Input: part model. Units: mm. Frame: model coordinates. A direction names the side the tool comes from. Give positions to 0.01 mm unless a question says otherwise; leave off trailing zeros. Order: outer loops, then holes, each group sorted by start corner. A loop starts at its lowest first (then second) coordinate and runs counter-clockwise, first axis right, second up. Notation, with made-up numbers: (67, 77) - (93, 77) arc R19 ccw to (93, 86) - close; hole circle Ø10 at (79.25, 45). An arc over 180 degrees is marked (long way). Use a Markdown table: item, result.
Autodesk Inventor part; units mm, degrees
ref_plane "YZ Plane" through (0, 0, 0) normal (1, 0, 0) x (0, 1, 0)
ref_plane "XZ Plane" through (0, 0, 0) normal (0, 1, 0) x (-1, 0, 0)
ref_plane "XY Plane" through (0, 0, 0) normal (0, 0, 1) x (1, 0, 0)
sketch "Boceto1" plane through (0, 0, 0) normal (0, 0, 1) x (1, 0, 0)
  circle A0 centre (0, 0) radius 13.175
  line L0 (0, -18.175) -> (-16.175, -18.175)
  line L1 (-9.175, 18.175) -> (9.175, 18.175)
  line L2 (16.175, -18.175) -> (0, -18.175)
  line L3 (-19.175, 0) -> (-19.175, 8)
  line L4 (-19.175, 8) -> (-16.175, 8)
  line L5 (-19.175, 0) -> (-19.175, -8)
  line L6 (-19.175, -8) -> (-16.175, -8)
  line L7 (-16.175, -18.175) -> (-16.175, -8)
  line L8 (-16.175, 8) -> (-16.175, 11.175)
  line L9 (16.175, -8) -> (19.175, -8)
  line L10 (19.175, -8) -> (19.175, 8)
  line L11 (19.175, 8) -> (16.175, 8)
  line L12 (16.175, 11.175) -> (16.175, 8)
  line L13 (16.175, -8) -> (16.175, -18.175)
  arc A1 (-9.175, 18.175) -> (-16.175, 11.175) centre (-9.175, 11.175) ccw
  arc A2 (16.175, 11.175) -> (9.175, 18.175) centre (9.175, 11.175) ccw
  dimension "d12" = 7
  dimension "d15" = 32.35
  dimension "d16" = 29.35
  dimension "d17" = 8
  dimension "d18" = 10.175
extrude "Extrusión1" add sketch "Boceto1" along normal blind 3
properties part number "muñeca3"
1. Pin query (flat end, axial travel): pin 1 (1.5 mm diameter, centred on x = 12.5, z = 2.5, fed in from +Y); pin 2 (1 mm diameter, centred on y = -13.5, z = 0.5, fed in from -X) (3 decimals); pin 3 (1.5 mm diameter, centred on y = 10.5, z = 2, fed in from +X) (3 decimals). Return the tip coordinate at first contact, or that it passes through.
Response:
| item | result |
|---|---|
| pin 1 | stops at y = 17.68 |
| pin 2 | stops at x = -16.175 |
| pin 3 | stops at x = 16.175 |
2. Section query C-C (x = 0). Return loops of the section in (y, z) (3 decimals).
Response:
| item | result |
|---|---|
| outline | (-18.175, 0) - (-13.175, 0) - (-13.175, 3) - (-18.175, 3) - close; (13.175, 0) - (18.175, 0) - (18.175, 3) - (13.175, 3) - close |
3. Material intervals for line 1 along Y through (x, z) = (0, 1.75) (3 decimals); line 2 along X through (y, z) = (0.5, 1.1) (1 decimal); line 3 along Y through (x, z) = (17, 1.9), sorted ascending.
Response:
| item | result |
|---|---|
| line 1 | y = -18.175 to -13.175, 13.175 to 18.175 |
| line 2 | x = -19.2 to -13.2, 13.2 to 19.2 |
| line 3 | y = -8 to 8 |
4. Section query B-B (z = 2.1). Return loops of the section in (x, y) (3 decimals).
Response:
| item | result |
|---|---|
| outline | (-19.175, -8) - (-16.175, -8) - (-16.175, -18.175) - (16.175, -18.175) - (16.175, -8) - (19.175, -8) - (19.175, 8) - (16.175, 8) - (16.175, 11.175) arc R7 ccw to (9.175, 18.175) - (-9.175, 18.175) arc R7 ccw to (-16.175, 11.175) - (-16.175, 8) - (-19.175, 8) - close; hole circle Ø26.35 at (0, 0) |
5. Section query A-A (y = 0). Return loops of the section in (x, z) (3 decimals), then the cut area to 3 significant figures.
Response:
| item | result |
|---|---|
| outline | (-19.175, 0) - (-13.175, 0) - (-13.175, 3) - (-19.175, 3) - close; (13.175, 0) - (19.175, 0) - (19.175, 3) - (13.175, 3) - close |
| area | 36.0 mm^2 |
6. Section query D-D (x = 17). Return loops of the section in (y, z), then the cut area to 3 significant figures.
Response:
| item | result |
|---|---|
| outline | (-8, 0) - (8, 0) - (8, 3) - (-8, 3) - close |
| area | 48.0 mm^2 |
7. Mould query, pull axis X, two halves, no side actions, for faces 1 (the face through (-14.18, 16.07, 1.48)), 2 (the face through (18, -8, 1)), 3 (the face through (-2.86, 12.86, 1.48)), 4 (the face through (19.175, 0, 1)). Classes: pulls with the +X half, pulls with the -X half, needs draft (parallel to the pull), parting line crosses it, or undercut.
Response:
| item | result |
|---|---|
| face 1 | pulls with the -X half |
| face 2 | needs draft |
| face 3 | undercut |
| face 4 | pulls with the +X half |
8. Set-up query: faces 5 (the face through (-18, -8, 1)), 6 (the face through (16.175, -13, 1)), 7 (the face through (-13, -4, 0)), 8 (the face through (-16.175, 10, 1)), 9 (the face through (16.175, 10, 1)). Return all of +Z, -Z, +X, -X, +Y, -Y with unobstructed straight access to the full face (end or side cutting, diameter ignored); none if empty.
Response:
| item | result |
|---|---|
| face 5 | +Z, -Z, -X, -Y |
| face 6 | +Z, -Z, +X, -Y |
| face 7 | -Z, +X, -X, +Y, -Y |
| face 8 | +Z, -Z, -X, +Y |
| face 9 | +Z, -Z, +X, +Y |
